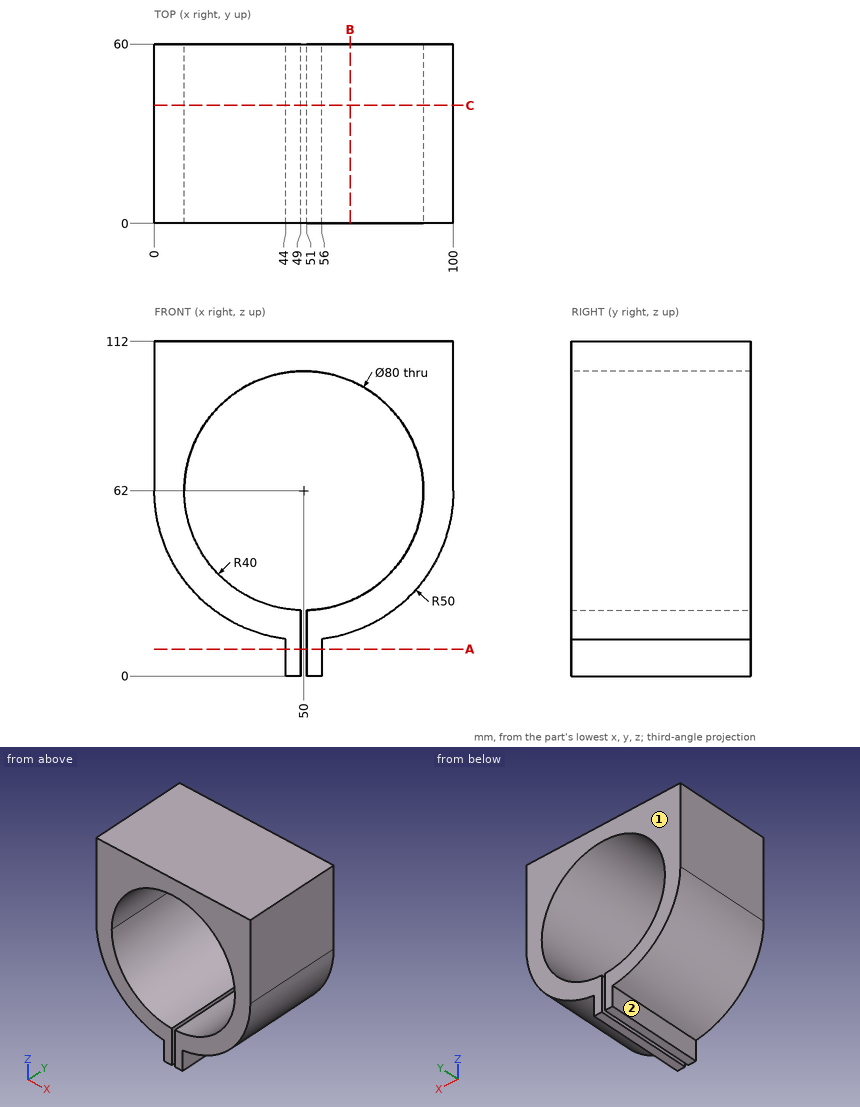
Job drawing, mm, ordinate dimensions from the low corner. One solid piece. A direction names the side the tool comes from. Round coordinates to 2 decimals unless told otherwise and drop trailing zeros. Loops run counter-clockwise (first coordinate to the right, second up) from the corner with the lowest first, then second, coordinate; pieces in that order, holes last. Notation, with made-up numbers: (-25, 60.25) -> (-1, 60.25) arc R21 cw to (-1, 67.25) -> close; hole circle Ø3 at (24.5, 68). An arc over 180 degrees is marked (long way). One line per item, written item: value. Start each with the question number.
Q1. Probe line 1 along X through (y, z) = (18, 62); line 2 along Z through (x, y) = (73.5, 21.5); line 3 along Z through (x, y) = (50, 35). List the from-to ranges inside material, lowest first.
Q2. 3-axis set-ups, long thin cutter, end or side, ignore diameter. For the marked faces 1 and 2: which of +Z, -Z, +X, -X, +Y, -Y reach the whole face in a straight line?
Q3. Cut at B-B on x = 65.5. List the corners of the cut face in (y, z).
Q4. Cut at A-A on z = 9. List the corners of the cut face in (x, y).
Q5. Cut at C-C on y = 39.5. List the corners of the cut face in (x, z).
Q6. Drop flat-ended pins along their axis: pin 1 Ø24 at (y, z) = (31, 7.5) entering from -X; pin 2 Ø17.5 at (y, z) = (29.5, 13) entering from +X; pin 3 Ø3.5 at (y, z) = (27.5, 7) entering from +X. Give the stop position or say it passes through.
Computed:
1. line 1: 0 to 10, 90 to 100
1. line 2: 17.87 to 29.63, 94.37 to 112
1. line 3: 102 to 112
2. face 1: +Z, -Z, +X, -X, +Y
2. face 2: -Z, -X, +Y, -Y
3. outline: (0, 14.46) -> (60, 14.46) -> (60, 25.13) -> (0, 25.13) -> close; (0, 98.87) -> (60, 98.87) -> (60, 112) -> (0, 112) -> close
4. outline: (44, 0) -> (49, 0) -> (49, 60) -> (44, 60) -> close; (51, 0) -> (56, 0) -> (56, 60) -> (51, 60) -> close
5. outline: (0, 62) arc R50 ccw to (44, 12.36) -> (44, 0) -> (49, 0) -> (49, 22.01) arc R40 cw (long way) to (51, 22.01) -> (51, 0) -> (56, 0) -> (56, 12.36) arc R50 ccw to (100, 62) -> (100, 112) -> (0, 112) -> close
6. pin 1: x = 23.66
6. pin 2: x = 79.66
6. pin 3: x = 56
